Source: three-view drawing plus pictorial views. Frame: mm from the lowest corner of the part. A direction names the side the tool comes from. Give positions to 0.01 mm unless a question says otherwise; leave off trailing zeros. Loops run counter-clockwise (first coordinate to the right, second up) from the corner with the lowest first, then second, coordinate; pieces in that order, holes last. Notation, with made-up numbers: (26.25, -37) -> (51.25, -37) arc R23 cw to (51.25, -7) -> close; hole circle Ø10 at (63.5, 14.5). An arc over 180 degrees is marked (long way). One line per item, written item: value. Start each with the question number.
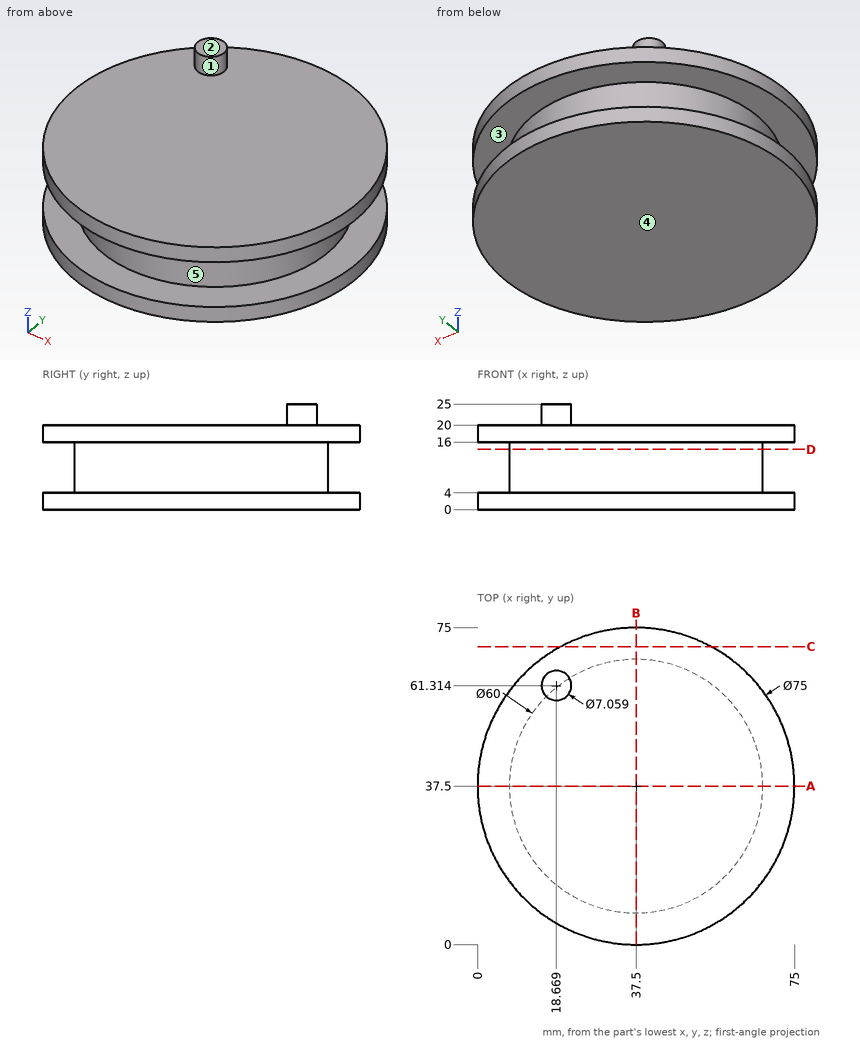
Item 1: Section D-D, the plane z = 14.25. Output: boundary loops of the cut face in (x, y), then the cut area to 3 significant figures.
Item 2: Ray query, line 1 along Z through (x, y) = (10, 53); line 2 along Z through (x, y) = (32, 36.5); line 3 along X through (y, z) = (43, 13). Return the intervals inside material, ascending. Write a range as [from, to].
Item 3: Section C-C, the plane y = 70.5. Output: boundary loops of the cut face in (x, z), then the cut area to 3 significant figures.
Item 4: Mould query, pull axis Z, two halves, no side actions, for the marked faces 1, 2 and 3. Classes: pulls with the +Z half, pulls with the -Z half, needs draft (parallel to the pull), parting line crosses it, or undercut.
Item 5: Pin query (flat end, axial travel): pin 1 (2 mm diameter, centred on x = 44.5, y = 59, fed in from +Z); pin 2 (1.5 mm diameter, centred on y = 57.5, z = 11.5, fed in from -X); pin 3 (1 mm diameter, centred on x = 25, z = 15, fed in from -Y) (1 decimal). Return the tip coordinate at first contact, or that it passes through.
Item 6: Section A-A, the plane y = 37.5. Output: boundary loops of the cut face in (x, z), then the cut area to 3 significant figures.
Item 7: Access query for the marked faces 4 and 5. Directions: +Z, -Z, +X, -X, +Y, -Y. A direction counts if a zero-diameter tool reaches every point of the face in a straight line with its end or side. Return the directions, or none.
Geometry check:
1. outline: circle Ø60 at (37.5, 37.5)
1. area: 2,830 mm2
2. line 1: z = [0, 4], [16, 20]
2. line 2: z = [0, 20]
2. line 3: x = [8.01, 66.99]
3. outline: (19.69, 0) -> (55.31, 0) -> (55.31, 4) -> (19.69, 4) -> close; (19.69, 16) -> (55.31, 16) -> (55.31, 20) -> (19.69, 20) -> close
3. area: 285 mm2
4. face 1: needs draft
4. face 2: pulls with the +Z half
4. face 3: undercut
5. pin 1: stops at z = 20
5. pin 2: stops at x = 14.49
5. pin 3: stops at y = 10
6. outline: (0, 0) -> (75, 0) -> (75, 4) -> (67.5, 4) -> (67.5, 16) -> (75, 16) -> (75, 20) -> (0, 20) -> (0, 16) -> (7.5, 16) -> (7.5, 4) -> (0, 4) -> close
6. area: 1,320 mm2
7. face 4: -Z, +X, -X, +Y, -Y
7. face 5: none
